Source: CAD feature listing. Evaluate the final solid. Frame: model axes, mm. A direction names the side the tool comes from. Give positions to 0.01 mm unless a question says otherwise; leave off trailing zeros. Loops run counter-clockwise (first coordinate to the right, second up) from the corner with the lowest first, then second, coordinate; pieces in that order, holes last. Notation, with made-up numbers: M 38,51 L 78,51 A17 ccw 78,74 Z; hole C 51,64.25 d9. An arc over 180 degrees is marked long. Answer in a Markdown table with one row per item.
Autodesk Inventor part; units mm, degrees
ref_plane "YZ Plane" through (0, 0, 0) normal (1, 0, 0) x (0, 1, 0)
ref_plane "XZ Plane" through (0, 0, 0) normal (0, 1, 0) x (-1, 0, 0)
ref_plane "XY Plane" through (0, 0, 0) normal (0, 0, 1) x (1, 0, 0)
sketch "Sketch1" plane through (0, 0, 0) normal (0, 0, 1) x (1, 0, 0)
  line L0 (-40, 35) -> (40, 35)
  line L1 (40, 35) -> (40, -35)
  line L2 (40, -35) -> (-40, -35)
  line L3 (-40, -35) -> (-40, 35)
  line L4 (-40, 35) -> (40, -35) construction
  line L5 (40, 35) -> (-40, -35) construction
  point P0 (0, 0)
  dimension "d0" = 70
  dimension "d1" = 80
extrude "Extrusion1" add sketch "Sketch1" along normal blind 30
sketch "Sketch2" plane through (-40, 35, 0) normal (0, 1, 0) x (1, 0, 0)
  line L0 (80, -30) -> (0, -30)
  circle A0 centre (80, -30) radius 25
  point P0 (40, 0)
  dimension "d4" = 50
extrude "Extrusion2" add sketch "Sketch2" against normal blind 70
extrude "Extrusion3" add sketch "Sketch2" along normal blind 0.5
sketch "Sketch3" plane through (-40, -35, 0) normal (0, -1, 0) x (1, 0, 0)
  circle A0 centre (79.901, 30.2944) radius 25
  line L0 (53.0517, 30.2944) -> (54.901, 30.2944)
  circle A1 centre (79.901, 30.2944) radius 24.5
  point P0 (40, 0)
  dimension "d9" = 50
  dimension "d19" = 49
fillet "Fillet1" radius 2 1 edges at (-40, 0, 30)
sketch "Sketch4" plane through (0, 0, 0) normal (0, 0, -1) x (-1, 0, 0)
  line L0 (40, -35) -> (38, -35)
  line L1 (40, -35) -> (39, -35)
  line L2 (-40, 35) -> (-15, 35)
  line L3 (-40, 35) -> (-39, 35)
  line L4 (39.5, -34.5) -> (-39.5, -34.5)
  line L5 (-39.5, -34.5) -> (-39.5, 34.5)
  line L6 (-39.5, 34.5) -> (39.5, 34.5)
  line L7 (39.5, 34.5) -> (39.5, -34.5)
  line L8 (40, -35) -> (40, 35)
  line L9 (-40, 35) -> (-40, -35)
  line L10 (-40, -35) -> (40, -35)
  line L11 (40, 35) -> (-40, 35)
  point P0 (0, 0)
  dimension "d24" = 0.5
  dimension "d25" = 0.5
  dimension "d26" = 0.5
  dimension "d27" = 0.5
extrude "Extrusion6" cut sketch "Sketch3" against normal blind 70 contours A1
sketch "Sketch5" plane through (-40, -35, 0) normal (0, -1, 0) x (1, 0, 0)
  arc A0 (80, 5) -> (55, 30) centre (80, 30) ccw
  circle A1 centre (80, 30) radius 25
  point P0 (40, 0)
extrude "Extrusion7" add sketch "Sketch5" along normal blind 0.5
extrude "Extrusion8" cut sketch "Sketch4" against normal blind 29.5 contours L4 L5 L6 L7
equation "\"BendRadius\" = Thickness"
equation "\"BendReliefWidth\" = Thickness"
equation "\"BendReliefDepth\" = 0.5 * Thickness"
equation "\"CornerReliefSize\" = 4 * Thickness"
equation "\"MinimumRemnant\" = 2 * Thickness"
equation "\"TransitionRadius\" = BendRadius"
equation "\"JacobiRadiusSize\" = Thickness"
equation "\"GapSize\" = Thickness"
properties part number "Battery Box" material "Steel, Mild"
Q1. Section query D-D (x = 0.5). Output: boundary loops of the cut face in (y, z).
Values follow:
| item | result |
|---|---|
| outline | M -35,0 L -34.5,0 L -34.5,29.5 L 34.5,29.5 L 34.5,0 L 35,0 L 35,30 L -35,30 Z |
Q2. Contact query for flat-ended pins moving along their axis: pin 1 Ø9 at (x, z) = (14, 10) entering from +Y; pin 2 Ø14.5 at (y, z) = (9, 16.5) entering from +X; pin 3 Ø1 at (x, y) = (34, -27.5) entering from +Z. Output: stop coordinate, or through.
Values follow:
| item | result |
|---|---|
| pin 1 | y = 35 |
| pin 2 | x = 64.21 |
| pin 3 | z = 54.39 |
Q3. Section query B-B (z = 44). Output: boundary loops of the cut face in (x, y).
Values follow:
| item | result |
|---|---|
| outline | M 19.29,-35.5 L 60.71,-35.5 L 60.71,35.5 L 19.29,35.5 Z; hole M 19.59,-35 L 60.21,-35 L 60.21,35 L 19.59,35 Z |
Q4. Ray query, probe 1 along Y at (x, z) = (28, 44.5); probe 2 along Y at (x, z) = (12, 25.5); probe 3 along Z at (x, y) = (-1.5, -13). Return the intervals inside material, ascending. Write a range as from..to.
Values follow:
| item | result |
|---|---|
| probe 1 | -35.5..-35, 35..35.5 |
| probe 2 | -35..-34.5, 34.5..35 |
| probe 3 | 29.5..30 |
Q5. Section query C-C (x = 50). Output: boundary loops of the cut face in (y, z).
Values follow:
| item | result |
|---|---|
| outline | M -35.5,7.09 L 35.5,7.09 L 35.5,52.91 L -35.5,52.91 Z; hole M -35,7.97 L 35,7.97 L 35,52.62 L -35,52.62 Z |
Q6. Mould query, pull axis Z, two halves, no side actions, for faces 4 (the flat face through (40, -35, 31)), 5 (the flat face through (-8, 34.5, 15)), 6 (the flat face through (40, 35, 31)), 7 (the flat face through (-12, 0, 29.5)). Classes: +Z half, -Z half, draft (parallel to the pull), parting line (faces both ways), or undercut.
Values follow:
| item | result |
|---|---|
| face 4 | undercut |
| face 5 | draft |
| face 6 | undercut |
| face 7 | -Z half |
Q7. Section query A-A (y = -22). Output: boundary loops of the cut face in (x, z), plus the area to 3 significant figures.
Values follow:
| item | result |
|---|---|
| outline | M -40,0 L -39.5,0 L -39.5,29.32 A2 ccw -40,28 Z; M -39.32,29.5 L 15.41,29.5 A24.5 cw long 39.5,5.8 L 39.5,0 L 40,0 L 40,5 A25 ccw long 15,30 L -38,30 A2 ccw Z |
| area | 98.0 mm^2 |
Q8. Reachability of faces 1 (the flat face through (-39.5, 0, 14)), 2 (the flat face through (-9, 35, 15)), 3 (the flat face through (39.5, 0, 3)) from +Z, -Z, +X, -X, +Y, -Y: full face, straight path, thin tool, end or side. Return the list, or none.
Values follow:
| item | result |
|---|---|
| face 1 | +Z, -Z |
| face 2 | -Z, -X, +Y |
| face 3 | -Z |
